Can you work these out from the model? Positions are in its coordinate system, mm. A direction names the side the tool comes from. Coordinates: 2 decimals unless noted, no trailing zeros. Loops run counter-clockwise (first coordinate to the right, second up) from the corner with the lowest first, then second, coordinate; pieces in that order, holes last. Notation, with made-up numbers: (-9.5, 32) -> (-4.5, 32) arc R15 cw to (-4.5, 55) -> close; hole circle Ø4 at (79, 47.25). An arc over 180 degrees is marked (long way). Use one line per item in the form item = value. Start each with the question number.
(1) Imagine slicing it at C-C (y = 5.5). List the corners of the cut face in (x, z) for me.
(2) Imagine slicing it at D-D (x = 37.5). List the corners of the cut face in (y, z) for me, plus the area to 3 significant figures.
(3) Thinking about a two-plate mould opening in X: for faces 1 (the flat face through (21, 5, 0)), 2 (the flat face through (16.5, 5, -3)), 3 (the cylindrical face through (40.227, 4.93, -12.358)), 4 (the cylindrical face through (25.466, 4.93, -12.521)), which applies, released by +X, released by -X, zero draft, split by the parting line, or undercut?
(4) I need wall thicknesses on line 1 (X direction, y = 2.5, z = -12); line 2 (Z direction, x = 39, y = 8); line 3 (X direction, y = 9, z = -10.75). Which ranges of each line are inside material? Lowest first, please. Write a range as [from, to].
(5) Imagine slicing it at A-A (z = -12). List the corners of the cut face in (x, y) for me, plus the area to 3 significant figures.
(6) Imagine slicing it at B-B (x = 21.5). List the corners of the cut face in (y, z) for me, plus the area to 3 significant figures.
(7) On a 3-axis mill with a long thin cutter (end or side, diameter ignored), from which of +Z, -Z, +X, -X, +Y, -Y can I reach the whole of each face in a straight line? I mean faces 5 (the flat face through (22, 5, -24)), 6 (the flat face through (26.5, 5, -3)). Say none if no direction works.
(8) I'm going to push flat-ended pins straight in: pin 1 (1.8 mm diameter, centred on y = 7, z = -2, fed in from -X); pin 2 (1.8 mm diameter, centred on y = 6.5, z = -1.5, fed in from +X). Where does each tip first touch, or does it pass through?
```python
from build123d import *

# Parameters (mm, degrees)
SKETCH_1_R      = 2.75
SKETCH_1_R_2    = 4
EXTRUDE_1_DEPTH = 10


with BuildPart() as part:
    # Эскиз1 → Бобышка-Вытянуть1 (new body)
    with BuildSketch(Plane(origin=(0, 0, 0), x_dir=(1, 0, 0), z_dir=(0, 1, 0))):
        Polygon((16.5, 0), (26.5, 0), (26.5, 6), (43, 8), (43, 17), (26.5, 24), (16.5, 24), (0, 17), (0, 8), (16.5, 6), align=None)
        with Locations(Location((5.5, 12, 0), (0, 0, 270))):
            Circle(SKETCH_1_R, mode=Mode.SUBTRACT)
        with Locations(Location((37.5, 12, 0), (0, 0, 270))):
            Circle(SKETCH_1_R, mode=Mode.SUBTRACT)
        with Locations(Location((21.5, 12, 0), (0, 0, 270))):
            Circle(SKETCH_1_R_2, mode=Mode.SUBTRACT)
    extrude(amount=EXTRUDE_1_DEPTH)


solid = part.part
```
Worked out:
q1.outline = (0, -17) -> (16.5, -24) -> (26.5, -24) -> (43, -17) -> (43, -8) -> (26.5, -6) -> (26.5, 0) -> (16.5, 0) -> (16.5, -6) -> (0, -8) -> close; hole circle Ø5.5 at (5.5, -12); hole circle Ø8 at (21.5, -12); hole circle Ø5.5 at (37.5, -12)
q2.outline = (0, -19.33) -> (10, -19.33) -> (10, -14.75) -> (0, -14.75) -> close; (0, -9.25) -> (10, -9.25) -> (10, -7.33) -> (0, -7.33) -> close
q2.area = 65.0 mm2
q3.face_1 = zero draft
q3.face_2 = released by -X
q3.face_3 = undercut
q3.face_4 = undercut
q4.line_1 = [0, 2.75], [8.25, 17.5], [25.5, 34.75], [40.25, 43]
q4.line_2 = [-18.7, -14.3], [-9.7, -7.52]
q4.line_3 = [0, 3.05], [7.95, 17.7], [25.3, 35.05], [39.95, 43]
q5.outline = (0, 0) -> (2.75, 0) -> (2.75, 10) -> (0, 10) -> close; (8.25, 0) -> (17.5, 0) -> (17.5, 10) -> (8.25, 10) -> close; (25.5, 0) -> (34.75, 0) -> (34.75, 10) -> (25.5, 10) -> close; (40.25, 0) -> (43, 0) -> (43, 10) -> (40.25, 10) -> close
q5.area = 240 mm2
q6.outline = (0, -24) -> (10, -24) -> (10, -16) -> (0, -16) -> close; (0, -8) -> (10, -8) -> (10, 0) -> (0, 0) -> close
q6.area = 160 mm2
q7.face_5 = -Z, +X, -X, +Y, -Y
q7.face_6 = +Z, +X, +Y, -Y
q8.pin_1 = 16.5
q8.pin_2 = 26.5
